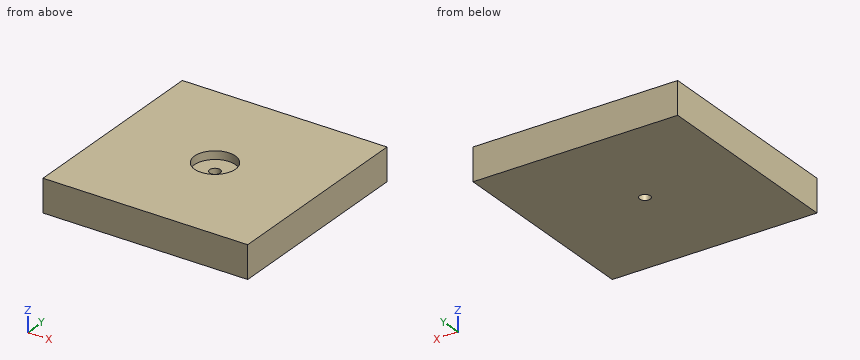
```python
from build123d import *

# Parameters (mm, degrees)
F0_W     = 50
F0_H     = 50
F1_DEPTH = 8
F2_R     = 5
F3_DEPTH = 2
F4_R     = 1.3
F5_DEPTH = 6.001


with BuildPart() as f1:
    # F0 (on Top) → F1 (new body)
    with BuildSketch(Plane.XY):
        Rectangle(F0_W, F0_H)
    extrude(amount=-F1_DEPTH)

    # F2 (on face) → F3 (cut)
    with BuildSketch(Plane.XY):
        Circle(F2_R)
    extrude(amount=-F3_DEPTH, mode=Mode.SUBTRACT)

    # F4 (on face) → F5 (cut, through all)
    with BuildSketch(Plane.XY.offset(-2)):
        Circle(F4_R)
    extrude(amount=-F5_DEPTH, mode=Mode.SUBTRACT)


solid = f1.part
```
Work out the finished part from the listing and answer in its coordinate system (mm). Coordinates: 2 decimals unless noted, no trailing zeros. Loops run counter-clockwise (first coordinate to the right, second up) from the corner with the lowest first, then second, coordinate; pieces in that order, holes last.
1) Section C-C (z = -0.75) is taken. Give the vertices of the cut face in (x, y).
Results:
outline: (-25, -25) - (25, -25) - (25, 25) - (-25, 25) - close; hole circle Ø10 at (0, 0)
2) Consider probe 1 along Y at (x, z) = (0, -4.85); probe 2 along Y at (x, z) = (0, -0.75); probe 3 along Z at (x, y) = (2.5, -0.5). Determine where each line is inside the solid, lowest interval first.
Results:
probe 1: y = -25 to -1.3, 1.3 to 25
probe 2: y = -25 to -5, 5 to 25
probe 3: z = -8 to -2
3) Section A-A (y = 0) is taken. Give the vertices of the cut face in (x, z).
Results:
outline: (-25, -8) - (-1.3, -8) - (-1.3, -2) - (-5, -2) - (-5, 0) - (-25, 0) - close; (1.3, -8) - (25, -8) - (25, 0) - (5, 0) - (5, -2) - (1.3, -2) - close
